Geometry: final body of the model. Coordinates: model frame, mm. A direction names the side the tool comes from. Give positions to 0.01 mm unless a question says otherwise; leave off trailing zeros. Write each loop counter-clockwise with the first axis right and the second up, starting at its lowest first coordinate (ties: lowest second). Pieces come first, ordered by that corner, then holes. Notation, with made-up numbers: (69.25, 26) - (113.25, 26) arc R22 cw to (113.25, 43) - close; hole circle Ø2 at (26, 73). An arc over 180 degrees is marked (long way). Use CSV: the item, a comma, the result in double quotes. Start each with the question number.
(1) Reachability of faces 5 (the flat face through (1, 25, 60)), 6 (the flat face through (77, 25, 52)), 7 (the flat face through (-14, 3, 3)), 8 (the flat face through (23, 25, 30)), 9 (the cylindrical face through (-14.383, 4.67, 1.479)) from +Z, -Z, +X, -X, +Y, -Y: full face, straight path, thin tool, end or side. Return the list, or none.
(2) Section A-A on x = -16. Output: boundary loops of the cut face in (y, z).
(3) Section C-C on x = 10. Output: boundary loops of the cut face in (y, z), and give its area (3 significant figures).
(4) Section B-B on z = 41. Output: boundary loops of the cut face in (x, y).
(5) Line query: probe 1 along Y at (x, z) = (-16, 4.3); probe 2 along Y at (x, z) = (16, 1); probe 3 along X at (y, z) = (5, 54). Output: solid intervals per line, ascending. Write a range as [from, to].
(6) First-contact query: pin 1 Ø10 at (x, z) = (60, 34.5) entering from +Y; pin 2 Ø3 at (y, z) = (6, 6.5) entering from -X; pin 3 Ø5 at (x, y) = (-54.5, 25.5) entering from -Z; pin 4 Ø21.5 at (y, z) = (28.5, 39.5) entering from +X. Flat tips, straight axial feed; report the tip coordinate or a pass-through.
(7) Draft query along Z for faces 1 (the flat face through (44.16, 24.65, 30.36)), 2 (the flat face through (-47.745, 24.65, 26.364)), 3 (the cylindrical face through (13.024, 1.718, 5.535)), 4 (the flat face through (-90, 25, 56)). Return one class per face: released by +Z, released by -Z, zero draft, split by the parting line, or undercut.
(8) Section D-D on y = 24. Output: boundary loops of the cut face in (x, z), and give its area (3 significant figures).
Solid Edge part; units mm, degrees
sketch "Sketch1" plane through (0, 0, 0) normal (0, -1, 0) x (1, 0, 0)
  line L0 (30, 0) -> (65, 52)
  line L1 (65, 52) -> (90, 52)
  line L2 (90, 52) -> (90, 60)
  line L3 (90, 60) -> (56.9204, 60)
  line L4 (56.9204, 60) -> (0, 60)
  line L5 (0, 60) -> (0, 52)
  line L6 (0, 52) -> (23, 52)
  line L7 (23, 52) -> (23, 8)
  line L8 (23, 8) -> (0, 8)
  line L9 (0, 8) -> (0, 0)
  line L10 (0, 0) -> (30, 0)
  dimension "D1" = 23
extrude "Protrusion1" add sketch "Sketch1" against normal blind 50
mirror "Mirror1" about plane through (0, 25, 4) normal (-1, 0, 0) of "Protrusion1"
sketch "Sketch2" plane through (0, 0, 26) normal (0, -1, 0) x (1, 0, 0)
  line L0 (30, -16.6796) -> (58.7267, 26)
  line L1 (58.7267, 26) -> (30, 26)
  line L2 (30, 26) -> (30, -16.6796)
extrude "Cutout1" cut sketch "Sketch2" against normal through all
sketch "Sketch3" plane through (0, 25, 0) normal (0, 0, -1) x (1, 0, 0)
  circle A0 centre (-16, 21) radius 1.75
  circle A1 centre (16, 21) radius 1.75
  circle A2 centre (16, -21) radius 1.75
  circle A3 centre (-16, -21) radius 1.75
extrude "Cutout2" cut sketch "Sketch3" against normal up to next
sketch "Sketch4" plane through (0, 25, 8) normal (0, 0, 1) x (1, 0, 0)
  circle A0 centre (-16, -21) radius 3.75
  circle A1 centre (16, -21) radius 3.75
  circle A2 centre (-16, 21) radius 3.75
  circle A3 centre (16, 21) radius 3.75
extrude "Extrusionsausschnitt_4" cut sketch "Sketch4" against normal blind 5
sketch "Sketch5" plane through (0, 25, 60) normal (0, 0, 1) x (-1, 0, 0)
  circle A0 centre (-62.5, 20) radius 1.4
  circle A1 centre (-62.5, -20) radius 1.4
  circle A2 centre (62.5, -20) radius 1.4
  circle A3 centre (62.5, 20) radius 1.4
  dimension "D1" = 62.5
  dimension "D2" = 62.5
extrude "Cutout3" cut sketch "Sketch5" against normal through all
mirror "Mirror2" about plane through (0, 0, 0) normal (1, 0, 0) of "Cutout1"
properties material "Nylon, allgemein"
Check values:
1,face 5,"+Z, +X, -X, +Y, -Y"
1,face 6,"-Z, +X, +Y, -Y"
1,face 7,"none"
1,face 8,"+Y, -Y"
1,face 9,"-Z"
2,outline,"(0, 0) - (2.25, 0) - (2.25, 3) - (0.25, 3) - (0.25, 8) - (0, 8) - close; (0, 52) - (50, 52) - (50, 60) - (0, 60) - close; (5.75, 0) - (44.25, 0) - (44.25, 3) - (42.25, 3) - (42.25, 8) - (7.75, 8) - (7.75, 3) - (5.75, 3) - close; (47.75, 0) - (50, 0) - (50, 8) - (49.75, 8) - (49.75, 3) - (47.75, 3) - close"
3,outline,"(0, 0) - (50, 0) - (50, 8) - (0, 8) - close; (0, 52) - (50, 52) - (50, 60) - (0, 60) - close"
3,area,"800 mm²"
4,outline,"(-57.6, 0) - (-51.32, 0) - (-51.32, 50) - (-57.6, 50) - close; (-30, 0) - (-23, 0) - (-23, 50) - (-30, 50) - close; (23, 0) - (30, 0) - (30, 50) - (23, 50) - close; (51.32, 0) - (57.6, 0) - (57.6, 50) - (51.32, 50) - close"
5,probe 1,"y = [0, 0.25], [7.75, 42.25], [49.75, 50]"
5,probe 2,"y = [0, 2.25], [5.75, 44.25], [47.75, 50]"
5,probe 3,"x = [-90, -63.9], [-61.1, 61.1], [63.9, 90]"
6,pin 1,"passes through"
6,pin 2,"stops at x = -35.38"
6,pin 3,"stops at z = 32.69"
6,pin 4,"stops at x = 63.82"
7,face 1,"undercut"
7,face 2,"released by -Z"
7,face 3,"undercut"
7,face 4,"zero draft"
8,outline,"(-90, 52) - (-65, 52) - (-30, 0) - (30, 0) - (65, 52) - (90, 52) - (90, 60) - (-90, 60) - close; hole (-58.73, 52) - (-30, 9.32) - (-30, 52) - close; hole (-23, 8) - (23, 8) - (23, 52) - (-23, 52) - close; hole (30, 9.32) - (58.73, 52) - (30, 52) - close"
8,area,"3,130 mm²"
